Autodesk Inventor part; units mm, degrees
ref_plane "YZ Plane" through (0, 0, 0) normal (1, 0, 0) x (0, 1, 0)
ref_plane "XZ Plane" through (0, 0, 0) normal (0, 1, 0) x (-1, 0, 0)
ref_plane "XY Plane" through (0, 0, 0) normal (0, 0, 1) x (1, 0, 0)
sketch "Skizze1" plane through (0, 0, 0) normal (0, 0, 1) x (1, 0, 0)
  line L0 (0, 0) -> (4, 0)
  line L1 (4, 0) -> (4, 8)
  line L2 (4, 8) -> (0, 8)
  line L3 (0, 8) -> (0, 0)
  dimension "d0" = 4
  dimension "d1" = 8
extrude "Extrusion1" add sketch "Skizze1" against normal blind 8
sketch "Skizze12" plane through (4, 0, 0) normal (1, 0, 0) x (0, 0, -1)
  line L0 (0, 8) -> (0, 0)
  line L1 (0, 0) -> (3, 0)
  line L2 (3, 0) -> (3, 4)
  line L3 (3, 4) -> (0, 4)
  line L4 (0, 4) -> (0, 0)
  line L5 (8, 0) -> (5, 0)
  line L6 (5, 0) -> (5, 4)
  line L7 (5, 4) -> (8, 4)
  line L8 (8, 4) -> (8, 0)
  dimension "d45" = 4
  dimension "d46" = 4
  dimension "d47" = 3
  dimension "d48" = 3
extrude "Extrusion10" cut sketch "Skizze12" against normal blind 5
sketch "Skizze13" plane through (4, 0, -3) normal (0, 0, 1) x (1, 0, 0)
  circle A0 centre (-2, 2) radius 1.7
  line L0 (0, 0) -> (-4, 0)
  line L1 (0, 4) -> (0, 0)
  dimension "d51" = 3.4
  dimension "d52" = 2
  dimension "d53" = 2
extrude "Extrusion11" cut sketch "Skizze13" against normal blind 3
sketch "Skizze14" plane through (4, 8, 0) normal (1, 0, 0) x (0, 0, -1)
  circle A0 centre (4, -2) radius 1.5
  line L0 (0, -4) -> (0, 0)
  line L1 (0, -4) -> (3, -4)
  point P0 (0, -8)
  dimension "d56" = 3
  dimension "d57" = 4
  dimension "d58" = 2
extrude "Extrusion12" cut sketch "Skizze14" against normal blind 10
properties part number "kamerahaltung"
Part model, mm, in its own coordinate system. A direction names the side the tool comes from. Give positions to 0.01 mm unless a question says otherwise; leave off trailing zeros. Write each loop counter-clockwise with the first axis right and the second up, starting at its lowest first coordinate (ties: lowest second). Pieces come first, ordered by that corner, then holes. Notation, with made-up numbers: (38.5, -9.5) -> (67.5, -9.5) arc R21 ccw to (67.5, 9.5) -> close; hole circle Ø2 at (34, 2.25). An arc over 180 degrees is marked (long way). Put each result on its own line as item: value. Start each with the question number.
Item 1: Which spindle directions (+Z, -Z, +X, -X, +Y, -Y) get a long thin tool onto all of the face, cutting with end or side? Do faces 1 (the face through (2, 4, -6)), 2 (the face through (2, 4, -2)), 3 (the face through (2.028, 5.425, -5.386)). Say none if no direction does.
Item 2: Cut at C-C (x = 2). List the corners of the cut face in (y, z), then the cut area to 3 significant figures.
Item 3: Cut at B-B (z = -4). List the corners of the cut face in (x, y), then the cut area to 3 significant figures.
Item 4: Wall check: L1, parallel to Y at x = 2, z = -4.05; L2, parallel to Y at x = 2, z = -3.6; L3, parallel to Z at x = 3.5, y = 3. Give the ranges that are in metal, low to high. Write a range as [from, to].
Item 5: Cut at D-D (x = 2.8). List the corners of the cut face in (y, z), then the cut area to 3 significant figures.
Item 6: Cut at A-A (y = 6). List the corners of the cut face in (x, z).
Item 7: Pull direction X, two halves, no side cores. Call faces 4 (the face through (3.62, 2.51, -3.99)), 5 (the face through (4, 4, -4)), 6 (the face through (2, 8, -4)): pulls with the +X half, pulls with the -X half, needs draft (parallel to the pull), parting line crosses it, or undercut.
Item 8: Pin check, flat tip, straight feed: pin 1 Ø1.5 at (x, y) = (2, 1) entering from +Z. Stop position of the tip, or through.
Answer list:
1. face 1: -Z, +X, -X, -Y
1. face 2: +Z, +X, -X, -Y
1. face 3: +X, -X
2. outline: (0, -5) -> (0.3, -5) -> (0.3, -3) -> (0, -3) -> close; (3.7, -5) -> (4, -5) -> (4, -8) -> (8, -8) -> (8, 0) -> (4, 0) -> (4, -3) -> (3.7, -3) -> close; hole circle Ø3 at (6, -4)
2. area: 26.1 mm2
3. outline: (0, 0) -> (4, 0) -> (4, 4.5) -> (0, 4.5) -> close; (0, 7.5) -> (4, 7.5) -> (4, 8) -> (0, 8) -> close; hole circle Ø3.4 at (2, 2)
3. area: 10.9 mm2
4. L1: y = [0, 0.3], [3.7, 4.5], [7.5, 8]
4. L2: y = [0, 0.3], [3.7, 4.55], [7.45, 8]
4. L3: z = [-5, -3]
5. outline: (0, -5) -> (0.5, -5) -> (0.5, -3) -> (0, -3) -> close; (3.5, -5) -> (4, -5) -> (4, -8) -> (8, -8) -> (8, 0) -> (4, 0) -> (4, -3) -> (3.5, -3) -> close; hole circle Ø3 at (6, -4)
5. area: 26.9 mm2
6. outline: (0, -8) -> (4, -8) -> (4, -5.5) -> (0, -5.5) -> close; (0, -2.5) -> (4, -2.5) -> (4, 0) -> (0, 0) -> close
7. face 4: undercut
7. face 5: pulls with the +X half
7. face 6: needs draft
8. pin 1: stops at z = -3
